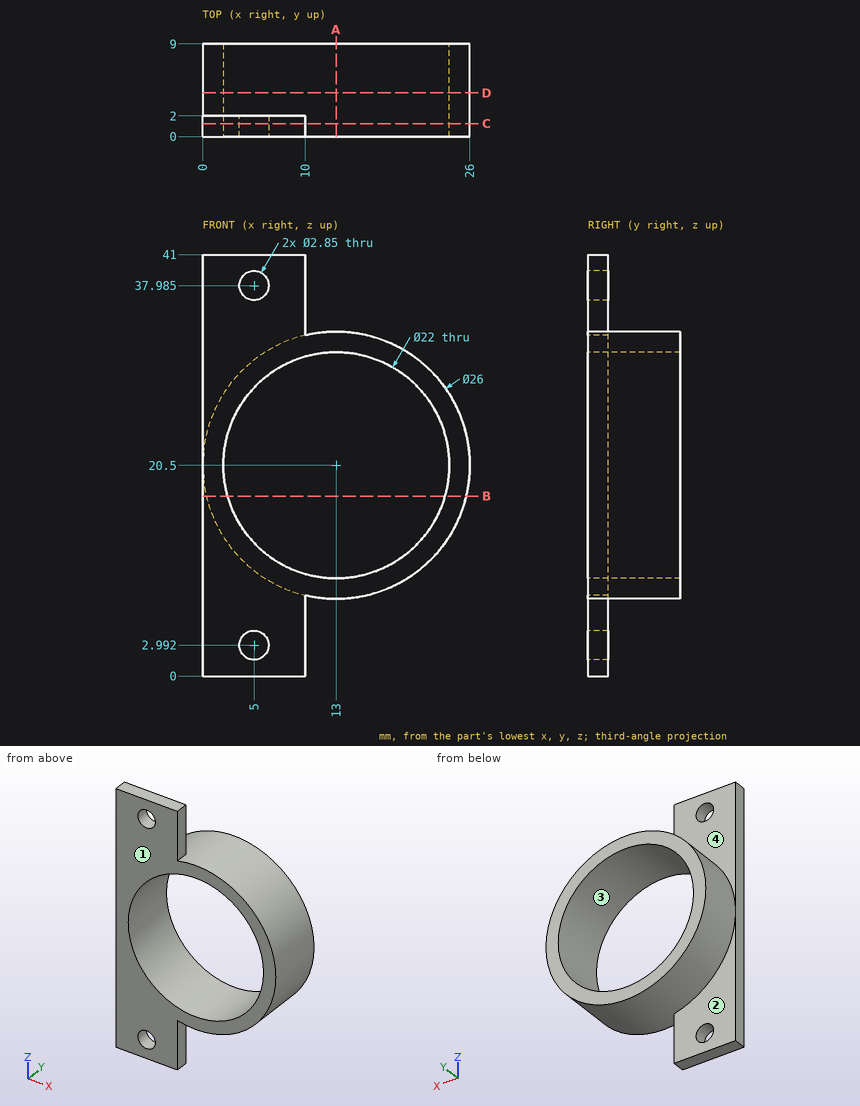
The figure shows three views and two pictorial views of one solid part (mm, origin at its lowest corner). Answer the questions. A direction names the side the tool comes from. Round coordinates to 2 decimals unless told otherwise and drop trailing zeros. Order: outer loops, then holes, each group sorted by start corner. A loop starts at its lowest first (then second) coordinate and runs counter-clockwise, first axis right, second up. Notation, with made-up numbers: M 54,16.25 L 92,16.25 A16 cw 92,28.25 Z; hole C 63.5,18.5 d1. An arc over 180 degrees is marked long. Put each result on its own line as item: value. Start each with the question number.
Q1. Section B-B, the plane z = 17.5 is taken. Write down the section's boundary in (x, y).
Q2. Flat-ended cylindrical pins translate along their axes: pin 1 (3 mm diameter, centred on y = 2, z = 24, fed in from +X) (1 decimal); pin 2 (2.5 mm diameter, centred on x = 5, z = 2.992, fed in from -Y); pin 3 (5 mm diameter, centred on x = 14, y = 5.5, fed in from +Z); pin 4 (0.6 mm diameter, centred on y = 1, z = 4, fed in from +X). Find the tip coordinate at first contact, or state that the pin passes through.
Q3. A tool of negligible diameter and unlimited length cuts with its end or side. For the marked faces 1 and 2, from which of +Z, -Z, +X, -X, +Y, -Y can it reach the whole face along a straight path? Write none if from no direction.
Q4. Section C-C, the plane y = 1.25 is taken. Give the number of separate pieces and of enclosed holes in the cut face, and give its area (3 significant figures).
Q5. For a pull along X with two mould halves and no side action, classify the marked faces 3 and 4 as pulls with the +X half, pulls with the -X half, needs draft (parallel to the pull), parting line crosses it, or undercut.
Q6. Section D-D, the plane y = 4.25 is taken. Write down the section's boundary in (x, z).
Q7. Section A-A, the plane x = 13 is taken. Write down the section's boundary in (y, z).
Q8. Straight lines are drawn through the part: L1, parallel to Y at x = 6.5, z = 6; L2, parallel to X at y = 1, z = 24; L3, parallel to Z at x = 13, y = 6. For each, find the intervals that lie inside material, in ascending order. Write a range as [from, to].
Findings below:
1. outline: M 0,0 L 2.42,0 L 2.42,9 L 0.35,9 L 0.35,2 L 0,2 Z; M 23.58,0 L 25.65,0 L 25.65,9 L 23.58,9 Z
2. pin 1: stops at x = 25.8
2. pin 2: passes through
2. pin 3: stops at z = 33.5
2. pin 4: stops at x = 10
3. face 1: +Z, -Z, +X, -X, -Y
3. face 2: -Z, -X, +Y
4. separate pieces: 1
4. enclosed holes: 3
4. area: 360 mm^2
5. face 3: undercut
5. face 4: needs draft
6. outline: C 13,20.5 d26; hole C 13,20.5 d22
7. outline: M 0,7.5 L 9,7.5 L 9,9.5 L 0,9.5 Z; M 0,31.5 L 9,31.5 L 9,33.5 L 0,33.5 Z
8. L1: y = [0, 2]
8. L2: x = [0, 2.57], [23.43, 25.52]
8. L3: z = [7.5, 9.5], [31.5, 33.5]
